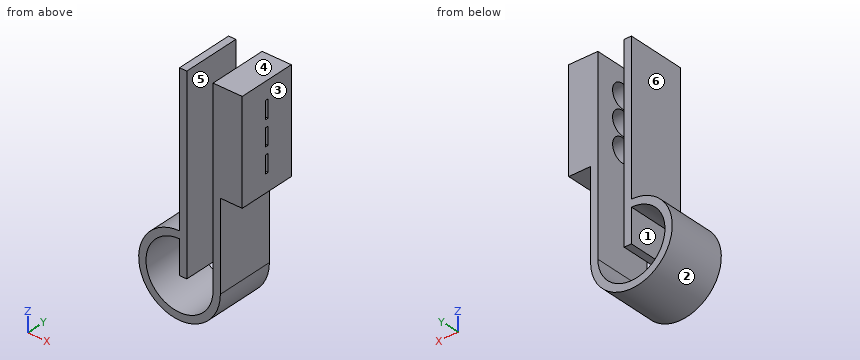
from build123d import *

# Parameters (mm, degrees)
BOSS_EXTRUDE1_DEPTH = 20
SKETCH2_R           = 4
CUT_EXTRUDE2_DEPTH  = 8
CUT_EXTRUDE4_DEPTH  = 10
SKETCH6_W           = 2.5
SKETCH6_H           = 20
SKETCH6_W_2         = 10
BOSS_EXTRUDE3_DEPTH = 5


with BuildPart() as part:
    # Sketch1 → Boss-Extrude1 (new body)
    with BuildSketch(Plane(origin=(0, 0, 0), x_dir=(1, 0, 0), z_dir=(0, 1, 0))):
        with BuildLine():
            Line((-29.801242739, -7.293134051), (-29.801242739, 22.74889672))
            ThreePointArc((-29.801242739, 22.74889672), (-53.700737675, 32.648391657), (-43.801242739, 8.74889672))
            Line((-43.801242739, 8.74889672), (-43.801242739, -37.25110328))
            Line((-43.801242739, -37.25110328), (-41.301242739, -37.25110328))
            Line((-41.301242739, -37.25110328), (-41.301242739, 22.74889672))
            Line((-41.301242739, 22.74889672), (-43.801242739, 22.74889672))
            Line((-43.801242739, 22.74889672), (-43.801242739, 11.24889672))
            ThreePointArc((-43.801242739, 11.24889672), (-51.932970722, 30.880624704), (-32.301242739, 22.74889672))
            Line((-32.301242739, 22.74889672), (-32.301242739, -37.25110328))
            Line((-32.301242739, -37.25110328), (-22.301242739, -37.25110328))
            Line((-22.301242739, -37.25110328), (-22.301242739, -7.25110328))
            Line((-22.301242739, -7.25110328), (-29.801242739, -7.293134051))
        make_face()
    extrude(amount=BOSS_EXTRUDE1_DEPTH)

    # Sketch2 → Cut-Extrude2 (cut)
    with BuildSketch(Plane.ZY.offset(32.301242739)):
        with Locations((16.25110328, 10)):
            Circle(SKETCH2_R)
        with Locations((33.20110328, 10)):
            Circle(SKETCH2_R)
        with Locations((24.75110328, 10)):
            Circle(SKETCH2_R)
    extrude(amount=-CUT_EXTRUDE2_DEPTH, mode=Mode.SUBTRACT)

    # Sketch3 → Cut-Extrude4 (cut)
    with BuildSketch(Plane(origin=(-22.301242739, 0, 0), x_dir=(0, 0, -1), z_dir=(1, 0, 0))):
        Polygon((-24.75110328, 10), (-27.75110328, 10.5), (-27.75110328, 9.5), align=None)
        Polygon((-21.75110328, 10.5), (-27.75110328, 10.5), (-24.75110328, 10), align=None)
        Polygon((-21.75110328, 10.5), (-24.75110328, 10), (-21.75110328, 9.5), align=None)
        Polygon((-21.75110328, 9.5), (-24.75110328, 10), (-27.75110328, 9.5), align=None)
        Polygon((-16.25110328, 10), (-19.25110328, 10.5), (-19.25110328, 9.5), align=None)
        Polygon((-13.25110328, 10.5), (-16.25110328, 10), (-13.25110328, 9.5), align=None)
        Polygon((-13.25110328, 10.5), (-19.25110328, 10.5), (-16.25110328, 10), align=None)
        Polygon((-13.25110328, 9.5), (-16.25110328, 10), (-19.25110328, 9.5), align=None)
        Polygon((-30.25110328, 10.5), (-33.25110328, 10), (-30.25110328, 9.5), align=None)
        Polygon((-30.25110328, 10.5), (-36.25110328, 10.5), (-33.25110328, 10), align=None)
        Polygon((-33.25110328, 10), (-36.25110328, 10.5), (-36.25110328, 9.5), align=None)
        Polygon((-30.25110328, 9.5), (-33.25110328, 10), (-36.25110328, 9.5), align=None)
    extrude(amount=-CUT_EXTRUDE4_DEPTH, mode=Mode.SUBTRACT)

    # Sketch6 → Boss-Extrude3 (add)
    with BuildSketch(Plane.XY.offset(37.25110328)):
        with Locations((-42.551242739, 10)):
            Rectangle(SKETCH6_W, SKETCH6_H)
        with Locations((-27.301242739, 10)):
            Rectangle(SKETCH6_W_2, SKETCH6_H)
    extrude(amount=BOSS_EXTRUDE3_DEPTH)


solid = part.part
CAD build for the part. Positions are in the model's coordinates, mm. Face numbers are marked on the shaded views. A direction names the side the tool comes from. Round coordinates to 2 decimals unless told otherwise and drop trailing zeros. Loops run counter-clockwise (first coordinate to the right, second up) from the corner with the lowest first, then second, coordinate; pieces in that order, holes last. Notation, with made-up numbers: M 84,33.25 L 143,33.25 A20 ccw 143,65.25 Z; hole C 8,88.5 d1. An arc over 180 degrees is marked long. One line per question, with ' | ' between items. Start each with the question number.
Item 1: Two-plate mould, pull along X, no slides. Class the marked faces 1, 2 and 3: pulls with the +X half, pulls with the -X half, needs draft (parallel to the pull), parting line crosses it, or undercut.
Item 2: Cut at B-B, the plane y = 3.75. Write the cut outline in (x, z), plus the area to 3 significant figures.
Item 3: Pin check, flat tips, straight feed: pin 1 Ø9 at (y, z) = (10, 25.5) entering from -X; pin 2 Ø6 at (x, y) = (-47, 6.5) entering from +Z; pin 3 Ø0.8 at (x, y) = (-23, 10) entering from -Z; pin 4 Ø1 at (x, z) = (-46, -6.5) entering from -Y. Stop position of each tip, or through.
Item 4: Cut at A-A, the plane z = 10.5. Write the cut outline in (x, y), plus the area to 3 significant figures.
Item 5: Which spindle directions (+Z, -Z, +X, -X, +Y, -Y) get a long thin tool onto all of the face, cutting with end or side? Do the marked faces 4, 5 and 6. Say none if no direction does.
Item 6: Wall check: line 1 (X direction, y = 15, z = 26); line 2 (X direction, y = 9.25, z = 32); line 3 (X direction, y = 17.75, z = -18). Give the ranges that are in metal, low to high.
Item 7: Cut at D-D, the plane x = -38. Write the cut outline in (y, z), plus the area to 3 significant figures.
Item 8: Cut at C-C, the plane z = 35. Write the cut outline in (x, y), plus the area to 3 significant figures.
Responses:
1) face 1: undercut | face 2: parting line crosses it | face 3: pulls with the +X half
2) outline: M -43.8,-22.75 L -41.3,-22.75 L -41.3,42.25 L -43.8,42.25 L -43.8,-8.75 A14 ccw long -29.8,-22.75 L -29.8,7.29 L -22.3,7.25 L -22.3,42.25 L -32.3,42.25 L -32.3,-22.75 A11.5 cw long -43.8,-11.25 Z | area: 738 mm²
3) pin 1: stops at x = -43.8 | pin 2: stops at z = -8.75 | pin 3: stops at z = 7.25 | pin 4: passes through
4) outline: M -43.8,0 L -41.3,0 L -41.3,20 L -43.8,20 Z; M -32.3,0 L -22.3,0 L -22.3,20 L -32.3,20 Z | area: 250 mm²
5) face 4: +Z, +X, -X, +Y, -Y | face 5: +Z, +Y, -Y | face 6: +Z, -X, +Y, -Y
6) line 1: x = -43.8 to -41.3, -32.3 to -22.3 | line 2: x = -43.8 to -41.3, -24.3 to -22.3 | line 3: x = -56.97 to -54.27, -43.8 to -41.3, -32.3 to -29.8
7) outline: M 0,-35.49 L 20,-35.49 L 20,-32.68 L 0,-32.68 Z | area: 56.2 mm²
8) outline: M -43.8,0 L -41.3,0 L -41.3,20 L -43.8,20 Z; M -32.3,0 L -22.3,0 L -22.3,9.5 L -24.3,9.5 L -24.3,6.43 L -32.3,6.43 Z; M -32.3,13.57 L -24.3,13.57 L -24.3,10.5 L -22.3,10.5 L -22.3,20 L -32.3,20 Z | area: 191 mm²
